from build123d import *

# Parameters (mm, degrees)
SKETCH1_R                           = 7.5
BOSS_EXTRUDE1_DEPTH                 = 58
CUT_EXTRUDE1_DEPTH                  = 107.60206377
CUT_EXTRUDE1_DEPTH_BACK             = 10
SKETCH3_W                           = 30
SKETCH3_H                           = 53
CUT_EXTRUDE3_DEPTH                  = 107.60206377
CUT_EXTRUDE3_DIRECTION_2_REACH      = 108.602
CUT_EXTRUDE3_DIRECTION_2_END_RADIUS = 50
CUT_EXTRUDE4_DEPTH                  = 107.60206377
SKETCH8_R                           = 7
CUT_EXTRUDE5_DEPTH                  = 107.60206377
SKETCH10_R                          = 7.5
CUT_EXTRUDE6_DEPTH                  = 6
CUT_EXTRUDE7_DEPTH                  = 4
CUT_EXTRUDE9_START                  = -6
SKETCH12_R                          = 7.5
CUT_EXTRUDE9_DEPTH                  = 6
CUT_EXTRUDE10_START                 = -4
CUT_EXTRUDE10_DEPTH                 = 4


with BuildPart() as part:
    # Sketch1 → Boss-Extrude1 (new body)
    with BuildSketch(Plane(origin=(0, 0, 0), x_dir=(0, 0, -1), z_dir=(1, 0, 0))):
        with BuildLine():
            Line((0, 0), (65, 0))
            Line((65, 0), (80, 8.660254038))
            Line((80, 8.660254038), (80, 31.339745962))
            Line((80, 31.339745962), (65, 40))
            Line((65, 40), (36.66060556, 40))
            ThreePointArc((36.66060556, 40), (16.66060556, 35.82575695), (0, 24))
            Line((0, 24), (0, 0))
        make_face()
        with Locations(Location((34, 19, 0), (0, 0, 180))):
            Circle(SKETCH1_R, mode=Mode.SUBTRACT)
    extrude(amount=BOSS_EXTRUDE1_DEPTH)

    # Sketch3 → Cut-Extrude1 (cut, two sides: drawn at the far end of the back side and taken through both)
    with BuildSketch(Plane(origin=(0, 0, 0), x_dir=(1, 0, 0), z_dir=(0, 1, 0)).offset(-CUT_EXTRUDE1_DEPTH_BACK)):
        with Locations((29, 42.5)):
            Rectangle(SKETCH3_W, SKETCH3_H)
    extrude(amount=CUT_EXTRUDE1_DEPTH + CUT_EXTRUDE1_DEPTH_BACK, mode=Mode.SUBTRACT)

    # Sketch5 → Cut-Extrude3 (cut)
    with BuildSketch(Plane(origin=(0, 0, 0), x_dir=(1, 0, 0), z_dir=(0, 1, 0))):
        Polygon((29, 0), (29, 16), (14, 16), (8, 16), (8, 0), align=None)
        Polygon((44, 16), (29, 16), (29, 0), (50, 0), (50, 16), align=None)
    extrude(amount=-CUT_EXTRUDE3_DEPTH, mode=Mode.SUBTRACT)

    # Cut-Extrude3 direction 2: up to this cylinder (the profile starts inside it)
    cut_extrude3_direction_2_end = Plane(origin=(29, -10, -36.66060556), z_dir=(-1, 0, 0)) * Cylinder(CUT_EXTRUDE3_DIRECTION_2_END_RADIUS, 339.204, mode=Mode.PRIVATE)
    # Sketch5 → Cut-Extrude3 direction 2 (cut, up to the surface)
    with BuildSketch(Plane(origin=(0, 0, 0), x_dir=(1, 0, 0), z_dir=(0, 1, 0)), mode=Mode.PRIVATE) as cut_extrude3_direction_2_sk1:
        Polygon((29, 0), (29, 16), (14, 16), (8, 16), (8, 0), align=None)
    cut_extrude3_direction_2_tool1 = extrude(cut_extrude3_direction_2_sk1.sketch, amount=CUT_EXTRUDE3_DIRECTION_2_REACH, mode=Mode.PRIVATE) & cut_extrude3_direction_2_end
    add(cut_extrude3_direction_2_tool1.solids().sort_by_distance((18.5, 0, -8))[0], mode=Mode.SUBTRACT)
    # Sketch5 → Cut-Extrude3 direction 2 (cut, up to the surface)
    with BuildSketch(Plane(origin=(0, 0, 0), x_dir=(1, 0, 0), z_dir=(0, 1, 0)), mode=Mode.PRIVATE) as cut_extrude3_direction_2_sk2:
        Polygon((44, 16), (29, 16), (29, 0), (50, 0), (50, 16), align=None)
    cut_extrude3_direction_2_tool2 = extrude(cut_extrude3_direction_2_sk2.sketch, amount=CUT_EXTRUDE3_DIRECTION_2_REACH, mode=Mode.PRIVATE) & cut_extrude3_direction_2_end
    add(cut_extrude3_direction_2_tool2.solids().sort_by_distance((39.5, 0, -8))[0], mode=Mode.SUBTRACT)

    # Sketch7 → Cut-Extrude4 (cut, through all)
    with BuildSketch(Plane(origin=(0, 0, 0), x_dir=(1, 0, 0), z_dir=(0, 1, 0))):
        Polygon((0, 65.69666313), (14.30333687, 80), (0, 80), align=None)
        Polygon((58, 65.69666313), (43.69666313, 80), (58, 80), align=None)
    extrude(amount=CUT_EXTRUDE4_DEPTH, mode=Mode.SUBTRACT)

    # Sketch8 → Cut-Extrude5 (cut, through all)
    with BuildSketch(Plane(origin=(0, 0, -80), x_dir=(-1, 0, 0), z_dir=(0, 0, -1))):
        with Locations((-29, 20)):
            Circle(SKETCH8_R)
    extrude(amount=-CUT_EXTRUDE5_DEPTH, mode=Mode.SUBTRACT)

    # Sketch10 → Cut-Extrude6 (cut)
    with BuildSketch(Plane.ZY):
        with BuildLine():
            Line((-36.66060556, 38), (-63.69666313, 38))
            Line((-63.69666313, 38), (-63.69666313, 2))
            Line((-63.69666313, 2), (0, 2))
            Line((0, 2), (0, 20.98386677))
            ThreePointArc((0, 20.98386677), (-0.7236706, 21.820381922), (-1.466424222, 22.64))
            ThreePointArc((-1.466424222, 22.64), (-17.46060556, 33.992726672), (-36.66060556, 38))
        make_face()
        with Locations((-34, 19)):
            Circle(SKETCH10_R, mode=Mode.SUBTRACT)
    extrude(amount=-CUT_EXTRUDE6_DEPTH, mode=Mode.SUBTRACT)

    # Sketch11 → Cut-Extrude7 (cut)
    with BuildSketch(Plane.ZY.offset(-6)):
        with BuildLine():
            Line((-63.69666313, 2), (-63.69666313, 38))
            Line((-63.69666313, 38), (-36.66060556, 38))
            ThreePointArc((-36.66060556, 38), (-27.510864492, 37.119870951), (-18.69666313, 34.511759933))
            Line((-18.69666313, 34.511759933), (-18.69666313, 2))
            Line((-18.69666313, 2), (-63.69666313, 2))
        make_face()
    extrude(amount=-CUT_EXTRUDE7_DEPTH, mode=Mode.SUBTRACT)

    # Sketch12 → Cut-Extrude9 (cut)
    with BuildSketch(Plane(origin=(58, 0, 0), x_dir=(0, 0, -1), z_dir=(1, 0, 0)).offset(CUT_EXTRUDE9_START)):
        with BuildLine():
            Line((63.69666313, 38), (36.66060556, 38))
            ThreePointArc((36.66060556, 38), (17.817714076, 34.146862182), (2, 23.206060023))
            Line((2, 23.206060023), (0, 24))
            Line((0, 24), (0, 0))
            Line((0, 0), (2, 2))
            Line((2, 2), (63.69666313, 2))
            Line((63.69666313, 2), (63.69666313, 38))
        make_face()
        with Locations(Location((34, 19, 0), (0, 0, 180))):
            Circle(SKETCH12_R, mode=Mode.SUBTRACT)
    extrude(amount=CUT_EXTRUDE9_DEPTH, mode=Mode.SUBTRACT)

    # Sketch13 → Cut-Extrude10 (cut)
    with BuildSketch(Plane(origin=(52, 0, 0), x_dir=(0, 0, -1), z_dir=(1, 0, 0)).offset(CUT_EXTRUDE10_START)):
        with BuildLine():
            Line((18.69666313, 34.511759933), (18.69666313, 2))
            Line((18.69666313, 2), (63.69666313, 2))
            Line((63.69666313, 2), (63.69666313, 38))
            Line((63.69666313, 38), (36.66060556, 38))
            ThreePointArc((36.66060556, 38), (27.510864492, 37.119870951), (18.69666313, 34.511759933))
        make_face()
    extrude(amount=CUT_EXTRUDE10_DEPTH, mode=Mode.SUBTRACT)


solid = part.part
For this review, take the finished solid that the model builds, in its own axes (mm). A direction names the side the tool comes from. Coordinates: 2 decimals unless noted, no trailing zeros. Order: outer loops, then holes, each group sorted by start corner. A loop starts at its lowest first (then second) coordinate and runs counter-clockwise, first axis right, second up. Notation, with made-up numbers: (42, -2.75) - (76, -2.75) arc R24 ccw to (76, 15.25) - close; hole circle Ø3 at (-22, 53). An arc over 180 degrees is marked (long way). Use one line per item in the form item = value.
Q1. For faces 1 (the flat face through (44, 20, -42)), 2 (the flat face through (54.96, 23.6, -1.01)), 3 (the flat face through (48, 20, -46)), 4 (the flat face through (8, 18, -18.697)), list the 3-axis set-ups (+Z, -Z, +X, -X, +Y, -Y) from which the entire face can be reached by the end or side of a thin tool; tool diameter is ignored.
Checked values:
face_1 = +Z, +Y, -Y
face_2 = +Z, +X
face_3 = +X
face_4 = -X
Q2. For probe 1 along X at (y, z) = (34, -39.5); probe 2 along Z at (x, y) = (35, 30); probe 3 along Y at (x, z) = (51.5, -28), list the stretches that pass through material, from the lowest coordinate up. Write a range as from..to.
Checked values:
probe_1 = 10..14, 44..48
probe_2 = -80..-69
probe_3 = 0..2, 37.21..39.24
Q3. Consider section A-A (z = -50.5). Give the boundary of the cut face in (x, y).
Checked values:
outline = (0, 0) - (14, 0) - (14, 40) - (0, 40) - (0, 38) - (10, 38) - (10, 2) - (0, 2) - close; (44, 0) - (58, 0) - (58, 2) - (48, 2) - (48, 38) - (58, 38) - (58, 40) - (44, 40) - close
Q4. Draft analysis for pull direction Y (two halves, no side actions). For faces 5 (the cylindrical face through (52.46, 37.55, -21.2)), 6 (the cylindrical face through (25.77, 13.79, -74.58)), 7 (the flat face through (8, 14, -8)), 8 (the flat face through (28.594, 4.27, -72.395)), state which applies: +Y half, -Y half, draft (parallel to the pull), parting line (faces both ways), or undercut.
Checked values:
face_5 = +Y half
face_6 = undercut
face_7 = draft
face_8 = -Y half
Q5. Consider section B-B (x = 29). Give the boundary of the cut face in (y, z).
Checked values:
outline = (2.31, -69) - (8.66, -80) - (13, -80) - (13, -69) - close; (27, -80) - (31.34, -80) - (37.69, -69) - (27, -69) - close
Q6. Consider section C-C (z = -31.5). Give the boundary of the cut face in (x, y), then the cut area to 3 significant figures.
Checked values:
outline = (0, 0) - (14, 0) - (14, 11.93) - (10, 11.93) - (10, 2) - (0, 2) - close; (0, 37.72) - (10, 37.72) - (10, 26.07) - (14, 26.07) - (14, 39.73) - (0, 39.73) - close; (44, 0) - (58, 0) - (58, 2) - (48, 2) - (48, 11.93) - (44, 11.93) - close; (44, 26.07) - (48, 26.07) - (48, 37.72) - (58, 37.72) - (58, 39.73) - (44, 39.73) - close
area = 285 mm2
Q7. For P1, Ø8, axis at y = 11.5, z = -5, coming from the +X side; P2, Ø24, axis at y = 19, z = -34, coming from the +X side; P3, Ø3, axis at x = 50.5, y = 26, coming from the -Z side, all flat-tipped, find the tip position at first contact; note any pin that passes through.
Checked values:
P1 = 52
P2 = 48
P3 = -74.7
Q8. Consider section D-D (y = 20). Give the number of separate pieces and of enclosed holes in the cut face, then the cut area to 3 significant figures.
Checked values:
separate_pieces = 4
enclosed_holes = 0
area = 776 mm2
